For this review, take the finished solid that the model builds, in its own axes (mm). Face numbers are marked on the shaded views. Round coordinates to 2 decimals unless told otherwise and drop trailing zeros. Loops run counter-clockwise (first coordinate to the right, second up) from the corner with the lowest first, then second, coordinate; pieces in that order, holes last. Notation, with made-up numbers: M 65.25,22 L 97.25,22 A23 ccw 97.25,56 Z; hole C 48,-1 d2. An arc over 180 degrees is marked long. One line per question, with ' | ' between items. Start each with the question number.
1) For probe 1 along Y at (x, z) = (16.5, 0); probe 2 along Z at (x, y) = (25.25, -14); probe 3 along Y at (x, z) = (18.75, -15), list the stretches that pass through material, from the lowest coordinate up. Write a range as from..to.
2) We need section A-A (z = 0). Give the boundary of the cut face in (x, y) (3 decimals), and give its area (3 significant figures).
3) We need section C-C (x = 24.5). Give the boundary of the cut face in (y, z) (3 decimals), and give its area (3 significant figures).
4) Mouldability with a two-part tool opening along Y and no side actions: class the marked faces 1, 2 and 3 as pulls with the +Y half, pulls with the -Y half, needs draft (parallel to the pull), parting line crosses it, or undercut.
5) We need section B-B (x = 27.75). Give the boundary of the cut face in (y, z) (3 decimals).
6) For pin 1 Ø6 at (x, y) = (21.5, -22.5) entering from -Z; pin 2 Ø2 at (x, y) = (21.5, 16) entering from -Z; pin 3 Ø3 at (x, y) = (22.5, 23.5) entering from -Z, all flat-tipped, find the tip position at first contact; note any pin that passes through.
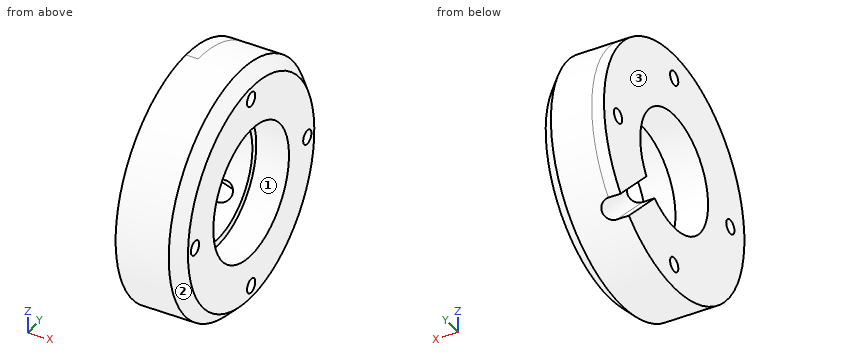
```python
from build123d import *

# Parameters (mm, degrees)
SKETCH_1_R           = 32
SKETCH_1_R_2         = 3
EXTRUDE_1_DEPTH      = 5
SKETCH_2_R           = 30
SKETCH_2_R_2         = 16.175
EXTRUDE_2_DEPTH      = 35
SKETCH_4_R           = 17
SKETCH_4_R_2         = 14
EXTRUDE_4_DEPTH      = 5
SKETCH_8_R           = 1.5
CUT_EXTRUDE_1_DEPTH  = 10
EXTRUDE_START        = 2
SKETCH_13_R          = 3.16745637
SKETCH_13_R_2        = 3
EXTRUDE_5_DEPTH      = 2
SKETCH_14_R          = 34.626760645
CUT_EXTRUDE_5_DEPTH  = 10
SKETCH_17_R          = 1.75
CUT_EXTRUDE_7_DEPTH  = 25
SKETCH_18_R          = 32
CUT_EXTRUDE_8_DEPTH  = 17
SKETCH_19_R          = 16.3
SKETCH_19_R_2        = 14.5
EXTRUDE_6_DEPTH      = 5
EXTRUDE_START_2      = 3
SKETCH_22_R          = 16.5
SKETCH_22_R_2        = 14.5
EXTRUDE_7_DEPTH      = 3
SKETCH_23_R          = 30
SKETCH_23_R_2        = 16.5
SKETCH_23_R_3        = 1.75
EXTRUDE_8_DEPTH      = 3
CHAMFER_2_SIZE       = 3
CUT_EXTRUDE_12_DEPTH = 52.961524227


with BuildPart() as part:
    # Эскиз1 → Бобышка-Вытянуть1 (new body)
    with BuildSketch(Plane(origin=(0, 0, 0), x_dir=(0, 0, -1), z_dir=(1, 0, 0))):
        Circle(SKETCH_1_R)
        with Locations((-24, 9)):
            Circle(SKETCH_1_R_2, mode=Mode.SUBTRACT)
        with Locations((-24, -9)):
            Circle(SKETCH_1_R_2, mode=Mode.SUBTRACT)
        with BuildLine():
            ThreePointArc((6.265686517, 10.234313483), (-12, 0), (6.265686517, -10.234313483))
            ThreePointArc((6.265686517, -10.234313483), (11.121320344, -11.121320344), (10.234313483, -6.265686517))
            ThreePointArc((10.234313483, -6.265686517), (12, 0), (10.234313483, 6.265686517))
            ThreePointArc((10.234313483, 6.265686517), (11.121320344, 11.121320344), (6.265686517, 10.234313483))
        make_face(mode=Mode.SUBTRACT)
    extrude(amount=EXTRUDE_1_DEPTH)

    # Эскиз2 → Бобышка-Вытянуть2 (add)
    with BuildSketch(Plane(origin=(5, 0, 0), x_dir=(0, 0, -1), z_dir=(1, 0, 0))):
        Circle(SKETCH_2_R)
        Circle(SKETCH_2_R_2, mode=Mode.SUBTRACT)
    extrude(amount=EXTRUDE_2_DEPTH)

    # Эскиз4 → Бобышка-Вытянуть4 (add)
    with BuildSketch(Plane(origin=(5, 0, 0), x_dir=(0, 0, -1), z_dir=(1, 0, 0))):
        Circle(SKETCH_4_R)
        with Locations(Location((0, 0, 0), (0, 0, 56.681914386))):
            Circle(SKETCH_4_R_2, mode=Mode.SUBTRACT)
    extrude(amount=EXTRUDE_4_DEPTH)

    # Эскиз8 → Вырез-Вытянуть1 (cut)
    with BuildSketch(Plane(origin=(5, 0, 0), x_dir=(0, 0, -1), z_dir=(1, 0, 0))):
        with Locations((-18, -20)):
            Circle(SKETCH_8_R)
        with Locations((18, -20)):
            Circle(SKETCH_8_R)
        with Locations((18, 20)):
            Circle(SKETCH_8_R)
        with Locations((-18, 20)):
            Circle(SKETCH_8_R)
    extrude(amount=-CUT_EXTRUDE_1_DEPTH, mode=Mode.SUBTRACT)

    # Эскиз13 → Бобышка-Вытянуть5 (add)
    with BuildSketch(Plane.ZY.offset(-5).offset(EXTRUDE_START)):
        with Locations((24, 9)):
            Circle(SKETCH_13_R)
        with Locations((24, -9)):
            Circle(SKETCH_13_R_2)
        with BuildLine():
            ThreePointArc((-6.121303477, 10.321319864), (-11.239729878, 11.239729878), (-10.321319864, 6.121303477))
            ThreePointArc((-10.321319864, 6.121303477), (-8.485281374, 8.485281374), (-6.121303477, 10.321319864))
        make_face()
        with BuildLine():
            ThreePointArc((-10.321319864, -6.121303477), (-11.239729878, -11.239729878), (-6.121303477, -10.321319864))
            ThreePointArc((-6.121303477, -10.321319864), (-8.485281374, -8.485281374), (-10.321319864, -6.121303477))
        make_face()
    extrude(amount=-EXTRUDE_5_DEPTH)

    # Эскиз14 → Вырез-Вытянуть5 (cut)
    with BuildSketch(Plane(origin=(40, 0, 0), x_dir=(0, 0, -1), z_dir=(1, 0, 0))):
        Circle(SKETCH_14_R)
    extrude(amount=-CUT_EXTRUDE_5_DEPTH, mode=Mode.SUBTRACT)

    # Эскиз17 → Вырез-Вытянуть7 (cut)
    with BuildSketch(Plane(origin=(30, 0, 0), x_dir=(0, 0, -1), z_dir=(1, 0, 0))):
        with Locations((-24, 0)):
            Circle(SKETCH_17_R)
        with Locations((0, 24)):
            Circle(SKETCH_17_R)
        with Locations((24, 0)):
            Circle(SKETCH_17_R)
        with Locations((0, -24)):
            Circle(SKETCH_17_R)
    extrude(amount=-CUT_EXTRUDE_7_DEPTH, mode=Mode.SUBTRACT)

    # Эскиз18 → Вырез-Вытянуть8 (cut)
    with BuildSketch(Plane.ZY):
        Circle(SKETCH_18_R)
    extrude(amount=-CUT_EXTRUDE_8_DEPTH, mode=Mode.SUBTRACT)

    # Эскиз19 → Бобышка-Вытянуть6 (add)
    with BuildSketch(Plane.ZY.offset(-17)):
        Circle(SKETCH_19_R)
        Circle(SKETCH_19_R_2, mode=Mode.SUBTRACT)
    extrude(amount=-EXTRUDE_6_DEPTH)

    # Эскиз22 → Бобышка-Вытянуть7 (add)
    with BuildSketch(Plane.ZY.offset(-17).offset(EXTRUDE_START_2)):
        Circle(SKETCH_22_R)
        Circle(SKETCH_22_R_2, mode=Mode.SUBTRACT)
    extrude(amount=-EXTRUDE_7_DEPTH)

    # Эскиз23 → Бобышка-Вытянуть8 (add)
    with BuildSketch(Plane.ZY.offset(-17)):
        Circle(SKETCH_23_R)
        Circle(SKETCH_23_R_2, mode=Mode.SUBTRACT)
        with Locations(Location((-24, 0, 0), (0, 0, 180))):
            Circle(SKETCH_23_R_3, mode=Mode.SUBTRACT)
        with Locations(Location((0, 24, 0), (0, 0, 180))):
            Circle(SKETCH_23_R_3, mode=Mode.SUBTRACT)
        with Locations(Location((24, 0, 0), (0, 0, 180))):
            Circle(SKETCH_23_R_3, mode=Mode.SUBTRACT)
        with Locations(Location((0, -24, 0), (0, 0, 180))):
            Circle(SKETCH_23_R_3, mode=Mode.SUBTRACT)
    extrude(amount=EXTRUDE_8_DEPTH)

    # Фаска2
    chamfer_2_edges = [part.edges().sort_by_distance(p)[0] for p in [
        (30, 0, 30),
    ]]
    chamfer(chamfer_2_edges, length=CHAMFER_2_SIZE)

    # Эскиз26 → Вырез-Вытянуть12 (cut, through all)
    with BuildSketch(Plane(origin=(0, 0, 0), x_dir=(1, 0, 0), z_dir=(0, -0.7071067811865437, 0.7071067811865513))):
        with BuildLine():
            Line((12, 2.5), (17, 2.5))
            ThreePointArc((17, 2.5), (19.5, 0), (17, -2.5))
            Line((17, -2.5), (12, -2.5))
            Line((12, -2.5), (12, 2.5))
        make_face()
    extrude(amount=-CUT_EXTRUDE_12_DEPTH, mode=Mode.SUBTRACT)


solid = part.part
```
Answers below:
1) probe 1: -30..-25.75, -22.25..-14.5, 14.5..22.25, 25.75..30 | probe 2: -26.53..-8.1, 8.1..26.53 | probe 3: -25.98..12.48, 17.52..25.98
2) outline: M 14,-30 L 27,-30 L 30,-27 L 30,-25.75 L 14,-25.75 Z; M 14,-22.25 L 30,-22.25 L 30,-16.175 L 22,-16.175 L 22,-14.5 L 14,-14.5 Z; M 14,14.5 L 22,14.5 L 22,16.175 L 30,16.175 L 30,22.25 L 14,22.25 Z; M 14,25.75 L 30,25.75 L 30,27 L 27,30 L 14,30 Z | area: 348 mm^2
3) outline: C 0,0 d60; hole C -24,0 d3.5; hole C 0,0 d32.35; hole C 0,-24 d3.5; hole C 0,24 d3.5; hole C 24,0 d3.5 | area: 1,970 mm^2
4) face 1: undercut | face 2: parting line crosses it | face 3: needs draft
5) outline: C 0,0 d58.5; hole C -24,0 d3.5; hole C 0,0 d32.35; hole C 0,-24 d3.5; hole C 0,24 d3.5; hole C 24,0 d3.5
6) pin 1: z = -22.8 | pin 2: z = -25.98 | pin 3: z = -20.4
